Design review of the part built by this model. Coordinates are the model's own, in mm. A direction names the side the tool comes from. Coordinates: 2 decimals unless noted, no trailing zeros. Loops run counter-clockwise (first coordinate to the right, second up) from the corner with the lowest first, then second, coordinate; pieces in that order, holes last. Notation, with made-up numbers: M 61.5,6 L 65.5,6 A15 ccw 65.5,17 Z; hole C 59.5,80.25 d8. An arc over 180 degrees is marked long. One line per item, written item: value.
```python
from build123d import *

# Parameters (mm, degrees)
F0_W     = 20
F0_H     = 31
F1_DEPTH = 44
F2_W     = 20
F2_H     = 10
F3_DEPTH = 10
F4_W     = 20
F4_H     = 10
F5_DEPTH = 30
F6_W     = 20
F6_H     = 10
F7_DEPTH = 30
F9_DEPTH = 20


with BuildPart() as f1:
    # F0 (on Top) → F1 (new body)
    with BuildSketch(Plane.XY):
        with Locations((10, 15.5)):
            Rectangle(F0_W, F0_H)
    extrude(amount=F1_DEPTH)

    # F2 (on face) → F3 (join)
    with BuildSketch(Plane.XY.offset(44)):
        with Locations((10, 26)):
            Rectangle(F2_W, F2_H)
        with Locations((10, 5)):
            Rectangle(F2_W, F2_H)
    extrude(amount=F3_DEPTH)

    # F4 (on face) → F5 (join)
    with BuildSketch(Plane.XZ):
        with Locations((10, 5)):
            Rectangle(F4_W, F4_H)
    extrude(amount=F5_DEPTH)

    # F6 (on face) → F7 (join)
    with BuildSketch(Plane(origin=(0, 31, 0), x_dir=(-1, 0, 0), z_dir=(0, 1, 0))):
        with Locations((-10, 5)):
            Rectangle(F6_W, F6_H)
    extrude(amount=F7_DEPTH)

    # F8 (on face) → F9 (cut)
    with BuildSketch(Plane.YZ.offset(20)):
        Polygon((-30, 1), (0, 10), (-30, 10), align=None)
        Polygon((31, 10), (61, 1), (61, 10), align=None)
    extrude(amount=-F9_DEPTH, mode=Mode.SUBTRACT)


solid = f1.part
```
(1) Tool access review of faces 1 (the flat face through (10, 10, 49)), 2 (the flat face through (10, 0, 32)), 3 (the flat face through (10, 31, 32)), 4 (the flat face through (20, 15, 21)): name each direction out of +Z, -Z, +X, -X, +Y, -Y from which nothing blocks a thin tool from reaching the whole face with its end or side.
Reply:
face 1: +Z, +X, -X
face 2: +Z, +X, -X, -Y
face 3: +Z, +X, -X, +Y
face 4: +Z, -Z, +X, +Y, -Y
(2) Mouldability with a two-part tool opening along Y and no side actions: class faces 5 (the flat face through (0, 15, 21)), 6 (the flat face through (10, 16, 44)), 7 (the flat face through (10.14, -15.21, 5.437)) as released by +Y, released by -Y, zero draft, split by the parting line, or undercut.
Reply:
face 5: zero draft
face 6: undercut
face 7: released by -Y
(3) We need section D-D on z = 38. State the section outline as (x, y) points, then the cut area to 3 significant figures.
Reply:
outline: M 0,0 L 20,0 L 20,31 L 0,31 Z
area: 620 mm2
(4) We need section B-B on x = 18.5. State the section outline as (y, z) points.
Reply:
outline: M -30,0 L 61,0 L 61,1 L 31,10 L 31,54 L 21,54 L 21,44 L 10,44 L 10,54 L 0,54 L 0,10 L -30,1 Z
(5) We need section C-C on y = 16. State the section outline as (x, z) points, then the cut area to 3 significant figures.
Reply:
outline: M 0,0 L 20,0 L 20,44 L 0,44 Z
area: 880 mm2
(6) Insertion check: pin 1 (2 mm diameter, centred on x = 12.5, z = 31.5, fed in from +Y); pin 2 (1.5 mm diameter, centred on x = 2.5, y = -3.5, fed in from +Z) (3 decimals); pin 3 (5 mm diameter, centred on x = 12.5, z = 46.5, fed in from -Y). Each pin has a flat end and moves straight along its axis. Give the tip position at first contact, or say it passes through.
Reply:
pin 1: stops at y = 31
pin 2: stops at z = 9.175
pin 3: stops at y = 0
(7) We need section A-A on z = 46. State the section outline as (x, y) points.
Reply:
outline: M 0,0 L 20,0 L 20,10 L 0,10 Z; M 0,21 L 20,21 L 20,31 L 0,31 Z
(8) To check wall thickness, follow line 1 along Y through (x, z) = (13.5, 14.5); line 2 along Y through (x, z) = (6.75, 49); line 3 along Z through (x, y) = (1.5, 18.5). State the ranges of each line that lie inside material, in increasing order. Write a range as [from, to].
Reply:
line 1: y = [0, 31]
line 2: y = [0, 10], [21, 31]
line 3: z = [0, 44]
